Design review of the part built by this model. Coordinates are the model's own, in mm. A direction names the side the tool comes from. Coordinates: 2 decimals unless noted, no trailing zeros. Write each loop counter-clockwise with the first axis right and the second up, starting at its lowest first coordinate (ties: lowest second). Pieces come first, ordered by that corner, then holes. Notation, with made-up numbers: (-1, 59) - (49, 59) arc R24 ccw to (49, 72) - close; hole circle Ø11 at (26, 61.25). An arc over 180 degrees is marked (long way). Answer as a JSON object with one key per item and string values.
Autodesk Inventor part; units mm, degrees
ref_plane "YZ Plane" through (0, 0, 0) normal (1, 0, 0) x (0, 1, 0)
ref_plane "XZ Plane" through (0, 0, 0) normal (0, 1, 0) x (-1, 0, 0)
ref_plane "XY Plane" through (0, 0, 0) normal (0, 0, 1) x (1, 0, 0)
sketch "Szkic1" plane through (0, 0, 0) normal (0, 1, 0) x (-1, 0, 0)
  circle A0 centre (2.6768, 3.8124) radius 6
  circle A1 centre (2.6768, 3.8124) radius 3
  point P0 (0, 0)
  dimension "d1" = 12
  dimension "d2" = 6
extrude "Wyciągnięcie proste1" add sketch "Szkic1" along normal blind 12
sketch "Szkic2" plane through (-2.6768, 12, 3.8124) normal (0, 1, 0) x (1, 0, 0)
  point P0 (2.6768, 3.8124)
sketch "Szkic4" plane through (-2.6768, 12, 3.8124) normal (0, 1, 0) x (1, 0, 0)
  circle A0 centre (0, 0) radius 6
  point P0 (2.6768, 3.8124)
  dimension "d5" = 12
extrude "Wyciągnięcie proste2" add sketch "Szkic4" along normal blind 5
sketch "Szkic5" plane through (-2.6768, 17, 3.8124) normal (0, 1, 0) x (1, 0, 0)
  circle A0 centre (0, 0) radius 6
  arc A1 (-0.78, 3.155) -> (-0.78, -3.155) centre (0, 0) ccw
  line L0 (-0.78, 4.55) -> (0.78, 4.55)
  line L1 (0.78, 4.55) -> (0.78, 3.155)
  line L2 (-0.78, -4.55) -> (0.78, -4.55)
  line L3 (0.78, -4.55) -> (0.78, -3.155)
  line L4 (-0.78, 3.155) -> (-0.78, 4.55)
  arc A2 (0.78, -3.155) -> (0.78, 3.155) centre (0, 0) ccw
  line L5 (-0.78, -3.155) -> (-0.78, -4.55)
  dimension "d8" = 12
  dimension "d10" = 1.56
  dimension "d12" = 1.56
extrude "Wyciągnięcie proste3" add sketch "Szkic5" along normal blind 8
properties part number "BlenderRoll"
(1) For pin 1 (1.5 mm diameter, centred on x = -2.5, z = 5, fed in from -Y); pin 2 (0.7 mm diameter, centred on y = 19.5, z = 0, fed in from -X); pin 3 (5 mm diameter, centred on x = -2.68, z = 3.81, fed in from +Y), all flat-tipped, find the tip position at first contact; note any pin that passes through.
Solved:
{"pin 1": "stops at y = 12", "pin 2": "stops at x = -7.58", "pin 3": "stops at y = 17"}
(2) Take a section at C-C, the plane y = 16. Write out the cut boundary in (x, z).
Solved:
{"outline": "circle Ø12 at (-2.68, 3.81)"}
(3) Tool access review of faces 3 (the face through (-1.897, 21, 0)), 4 (the face through (-4, 0, 7)), 5 (the face through (-0.3, 5.92, 5.64)): name each direction out of +Z, -Z, +X, -X, +Y, -Y from which nothing blocks a thin tool from reaching the whole face with its end or side.
Solved:
{"face 3": "+Y", "face 4": "+Z, -Z, +X, -X, -Y", "face 5": "-Y"}
(4) To check wall thickness, follow line 1 (Z direction, x = -2.5, y = 23.5) (3 decimals); line 2 (Y direction, x = -1.5, z = 2.5); line 3 (X direction, y = 10, z = 4). State the ranges of each line that lie inside material, in increasing order. Write a range as from..to.
Solved:
{"line 1": "z = -2.185..-0.738, 8.362..9.81", "line 2": "y = 12..17", "line 3": "x = -8.67..-5.67, 0.32..3.32"}
(5) Take a section at B-B, the plane y = 8.5. Write out the cut boundary in (x, z).
Solved:
{"outline": "circle Ø12 at (-2.68, 3.81); hole circle Ø6 at (-2.68, 3.81)"}
(6) The part is to be moulded in two halves that separate along X. For faces 1 (the face through (0, 25, 6)), 2 (the face through (-3, 21, 8.362)), say which applies: pulls with the +X half, pulls with the -X half, needs draft (parallel to the pull), parting line crosses it, or undercut.
Solved:
{"face 1": "needs draft", "face 2": "undercut"}
(7) Take a section at A-A, the plane y = 23. Write out the cut boundary in (x, z), and give its area (3 significant figures).
Solved:
{"outline": "circle Ø12 at (-2.68, 3.81); hole (-3.46, -0.74) - (-1.9, -0.74) - (-1.9, 0.66) arc R3.25 ccw to (-1.9, 6.97) - (-1.9, 8.36) - (-3.46, 8.36) - (-3.46, 6.97) arc R3.25 ccw to (-3.46, 0.66) - close", "area": "75.8 mm^2"}
